Read the model definition and answer for the solid it produces. Units are mm, in the model's axes. A direction names the side the tool comes from. Give positions to 0.01 mm unless a question says otherwise; leave off trailing zeros.
Item 1: Which of the six approach directions +Z, -Z, +X, -X, +Y, -Y give full straight-line access (tool end or side, diameter ignored) to faces 1 (the face through (-290.45, -3.78, -2.9)), 2 (the face through (-295.275, 0, 0)), 3 (the face through (290.45, -3.78, -2.9))?
Item 2: Find the intervals of material crossed by line 1 along X through (y, z) = (0, 20.5), in increasing order.
Item 3: Given pin 1 Ø8 at (y, z) = (7.5, 19) entering from +X; pin 2 Ø8 at (y, z) = (-6, 7.5) entering from -X; pin 3 Ø5.5 at (y, z) = (-3, -6.5) entering from +X (3 decimals), each flat-ended and moving along its own axis, determine where each tip first touches the part or whether it passes through.
from build123d import *

# Parameters (mm, degrees)
F0_W     = 19.05
F0_H     = 50.8
F1_DEPTH = 295.275
F3_W     = 73.66158
F3_H     = 70.153892
F3_R     = 4.7625
F4_DEPTH = 9.526
F6_W     = 59.882906
F6_H     = 61.81458
F6_R     = 4.7625
F7_DEPTH = 9.525


with BuildPart() as f1:
    # F0 (on Right) → F1 (new body, symmetric)
    with BuildSketch(Plane.YZ):
        Rectangle(F0_W, F0_H)
    extrude(amount=F1_DEPTH, both=True)

    # F3 (on offset) → F4 (cut, through all)
    with BuildSketch(Plane.YZ.offset(285.75)):
        Rectangle(F3_W, F3_H)
        Circle(F3_R, mode=Mode.SUBTRACT)
    extrude(amount=F4_DEPTH, mode=Mode.SUBTRACT)

    # F6 (on offset) → F7 (cut)
    with BuildSketch(Plane.YZ.offset(-285.75)):
        Rectangle(F6_W, F6_H)
        Circle(F6_R, mode=Mode.SUBTRACT)
    extrude(amount=-F7_DEPTH, mode=Mode.SUBTRACT)


solid = f1.part
Response values:
1. face 1: -X
1. face 2: +Z, -Z, -X, +Y, -Y
1. face 3: +X
2. line 1: x = -285.75 to 285.75
3. pin 1: stops at x = 285.75
3. pin 2: stops at x = -285.75
3. pin 3: stops at x = 295.275
